Part model, mm, in its own coordinate system. Give positions to 0.01 mm unless a question says otherwise; leave off trailing zeros. Order: outer loops, then holes, each group sorted by start corner. A loop starts at its lowest first (then second) coordinate and runs counter-clockwise, first axis right, second up. Notation, with made-up numbers: (-29.5, 5.5) - (10.5, 5.5) arc R14 ccw to (10.5, 30.5) - close; hole circle Ø10 at (16, 7). An arc over 180 degrees is marked (long way). One line per item, written item: value.
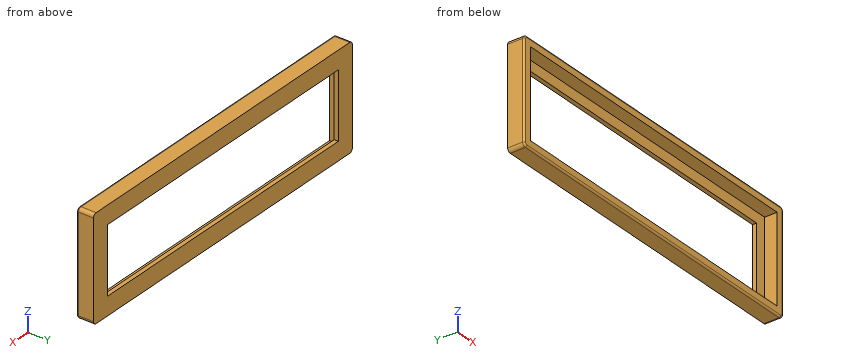
```python
from build123d import *

# Parameters (mm, degrees)
SKETCH051_W   = 100.7
SKETCH051_H   = 30.7
SKETCH051_W_2 = 89.8
SKETCH051_H_2 = 19.8
PAD022_DEPTH  = 1.25
SKETCH052_W   = 100.7
SKETCH052_H   = 30.7
SKETCH052_W_2 = 96
SKETCH052_H_2 = 26
PAD023_DEPTH  = 3.75
FILLET_R      = 1
FILLET005_R   = 0.5


with BuildPart() as part:
    # Sketch051 → Pad022 (new body)
    with BuildSketch(Plane.XZ):
        with Locations((0, 21.5)):
            Rectangle(SKETCH051_W, SKETCH051_H)
        with Locations((0, 21.5)):
            Rectangle(SKETCH051_W_2, SKETCH051_H_2, mode=Mode.SUBTRACT)
    extrude(amount=PAD022_DEPTH)

    # Sketch052 (on Face10 of Pad022) → Pad023 (join)
    with BuildSketch(Plane.XZ.offset(1.25)):
        with Locations((0, 21.5)):
            Rectangle(SKETCH052_W, SKETCH052_H)
        with Locations((0, 21.5)):
            Rectangle(SKETCH052_W_2, SKETCH052_H_2, mode=Mode.SUBTRACT)
    extrude(amount=PAD023_DEPTH)

    # Fillet
    fillet_edges = [part.edges().sort_by_distance(p)[0] for p in [
        (-50.35, -3.125, 36.85),
        (-50.35, -3.125, 6.15),
        (50.35, -3.125, 36.85),
        (50.35, -3.125, 6.15),
    ]]
    fillet(fillet_edges, radius=FILLET_R)

    # Fillet005
    fillet005_edges = [part.edges().sort_by_distance(p)[0] for p in [
        (0, -5, 6.15),
    ]]
    fillet(fillet005_edges, radius=FILLET005_R)


with BuildPart() as part_1:
    # Body011 placement: moved
    add(part.part.moved(Location((0, -70, 0))))


solid = part_1.part
```
1) Drill centre lines: line 1 along Z through (x, y) = (-14.5, -71.6); line 2 along X through (y, z) = (-74.2, 20); line 3 along X through (y, z) = (-70.55, 22). Where is each one in solid material? Low to high. Write a range as from..to.
Outcome:
line 1: z = 6.15..8.5, 34.5..36.85
line 2: x = -50.35..-48, 48..50.35
line 3: x = -50.35..-44.9, 44.9..50.35
2) Cut at B-B, the plane y = -72.35. Give the cut face in (x, z).
Outcome:
outline: (-50.35, 7.15) arc R1 ccw to (-49.35, 6.15) - (49.35, 6.15) arc R1 ccw to (50.35, 7.15) - (50.35, 35.85) arc R1 ccw to (49.35, 36.85) - (-49.35, 36.85) arc R1 ccw to (-50.35, 35.85) - close; hole (-48, 8.5) - (48, 8.5) - (48, 34.5) - (-48, 34.5) - close
3) Cut at D-D, the plane z = 9.5. Give the cut face in (x, y).
Outcome:
outline: (-50.35, -74.5) arc R0.5 ccw to (-49.85, -75) - (-48, -75) - (-48, -71.25) - (48, -71.25) - (48, -75) - (49.85, -75) arc R0.5 ccw to (50.35, -74.5) - (50.35, -70) - (-50.35, -70) - close
4) Cut at C-C, the plane z = 14.5. Give the cut face in (x, y), then the cut area to 3 significant figures.
Outcome:
outline: (-50.35, -74.5) arc R0.5 ccw to (-49.85, -75) - (-48, -75) - (-48, -71.25) - (-44.9, -71.25) - (-44.9, -70) - (-50.35, -70) - close; (44.9, -71.25) - (48, -71.25) - (48, -75) - (49.85, -75) arc R0.5 ccw to (50.35, -74.5) - (50.35, -70) - (44.9, -70) - close
area: 31.1 mm^2
5) Cut at A-A, the plane x = 19. Give the cut face in (y, z), then the cut area to 3 significant figures.
Outcome:
outline: (-75, 6.65) arc R0.5 ccw to (-74.5, 6.15) - (-70, 6.15) - (-70, 11.6) - (-71.25, 11.6) - (-71.25, 8.5) - (-75, 8.5) - close; (-75, 34.5) - (-71.25, 34.5) - (-71.25, 31.4) - (-70, 31.4) - (-70, 36.85) - (-74.5, 36.85) arc R0.5 ccw to (-75, 36.35) - close
area: 31.1 mm^2
